Autodesk Inventor part; units mm, degrees
ref_plane "Work Plane1" through (104.775, 0, 0) normal (0, 0, -1) x (1, 0, 0)
ref_plane "YZ Plane" through (0, 0, 0) normal (1, 0, 0) x (0, 1, 0)
ref_plane "XZ Plane" through (0, 0, 0) normal (0, 1, 0) x (-1, 0, 0)
sketch "Sketch1" plane through (0, 0, 0) normal (0, 0, 1) x (1, 0, 0)
  line L0 (15.875, 0) -> (15.875, 2.0828)
  line L1 (15.875, 2.0828) -> (4.8293, 2.0828)
  line L2 (4.8293, 2.0828) -> (2.8448, 2.0828)
  line L3 (0, 3.9497) -> (0, 1.3785)
  line L4 (0, 1.3785) -> (1.9304, 1.3785)
  line L5 (1.9304, 1.3785) -> (2.7263, 0)
  line L6 (2.7263, 0) -> (15.875, 0)
  line L7 (0, 3.9497) -> (0.6972, 3.9497)
  line L8 (0.6972, 3.9497) -> (2.8448, 2.0828)
  line L9 (2.8448, 2.0828) -> (2.8448, 2.0828)
  line L10 (4.8293, 2.0828) -> (2.8448, 2.0828) construction
  line L11 (2.8448, 2.0828) -> (2.8448, 2.0828)
  line L12 (-3.175, 0) -> (19.05, 0)
  line L13 (0, -0.7899) -> (0, 4.7396)
  dimension "d0" = 15.875
  dimension "d1" = 11.0457
  dimension "d2" = 1.9304
  dimension "d3" = 4.1656
  dimension "d6" = 2.8448
  dimension "d7" = 41
  dimension "d8" = 2.757
  dimension "d9" = 60
  dimension "d10" = 7.8994
  dimension "d11" = 4.1656
  dimension "d12" = 1.9845
revolve "Body" add sketch "Sketch1" angle 360 about axis through (2.7263, 0, 0) along (1, 0, 0) contours L6 L5 L4 L3 L7 L8 L2 L1 L0
sketch "Sketch2" plane through (0, 0, 0) normal (-1, 0, 0) x (0, 0, 1)
  circle A0 centre (0, 0) radius 1.3785
  line L0 (0, -5.5296) -> (0, 5.5296)
  line L1 (-5.5296, 0) -> (5.5296, 0)
  line L2 (1.3785, 0) -> (0.6892, -1.1938)
  line L3 (0.6892, -1.1938) -> (-0.6892, -1.1938)
  line L4 (-0.6892, -1.1938) -> (-1.3785, 0)
  line L5 (-1.3785, 0) -> (-0.6892, 1.1938)
  line L6 (-0.6892, 1.1938) -> (0.6892, 1.1938)
  line L7 (0.6892, 1.1938) -> (1.3785, 0)
  point P0 (0, 1.3785)
extrude "Slot" add sketch "Sketch2" against normal up to next contours L7 A0 | A0 L2 | L6 L0 A0 | A0 L0 L3 | L0 L6 A0 | A0 L3 L0 | L4 A0 | A0 L5
thread "Thread"
chamfer "Chamfer1" distance 0.4724 distance2 0.9449 1 edges at (15.875, -2.0828, 0) measured on face at (15.875, 0.3944, 0.7269)
ref_plane "Work Plane1" through (104.775, 0, 0) normal (0, 0, -1) x (1, 0, 0)
equation "\"d15\" = GEL"
equation "\"d17\" = -0.5 * SPD + 0.5 * GD"
equation "\"d18\" = GUL"
equation "\"d0\" = NLG"
equation "\"d1\" = GEL"
equation "\"d2\" = INTI"
equation "\"d3\" = GD"
equation "\"d6\" = KOH"
equation "\"d7\" = 0.5 * SEWI"
equation "\"d8\" = 1.1547 * SW"
equation "\"d10\" = KOD"
equation "\"d11\" = BDM"
equation "\"d12\" = GAL"
equation "\"NLG\" = 15.875"
equation "\"INTI\" = 1.9304"
equation "\"GEL\" = 11.0457"
equation "\"GAL\" = 1.9845"
equation "\"KOH\" = 2.8448"
equation "\"KOD\" = 7.8994"
equation "\"GUL\" = 0.94488"
equation "\"SPD\" = 3.22072"
equation "\"BDM\" = NND"
equation "\"GD\" = NND"
equation "\"SEWI\" = 82deg"
equation "\"SW\" = 2.3876"
equation "\"TOA\" = 30deg"
equation "\"GD1\" = SPD"
equation "\"THREADDIA\" = 4.1656"
equation "\"HHPTC\" = 0.79375"
equation "\"NND\" = 4.1656"
equation "\"E0\" = 1.155 * SW"
properties part number "ANSI B18.3 - 8-32 UNC x 0.625" material "Steel, Mild"
Input: part model. Units: mm. Frame: model coordinates. A direction names the side the tool comes from. Give positions to 0.01 mm unless a question says otherwise; leave off trailing zeros. Loops run counter-clockwise (first coordinate to the right, second up) from the corner with the lowest first, then second, coordinate; pieces in that order, holes last. Notation, with made-up numbers: M 57.5,61.25 L 90.5,61.25 A10 ccw 90.5,76.25 Z; hole C 22,86.25 d8. An arc over 180 degrees is marked long. Answer as CSV lines item,"result". Start each with the question number.
1. Section A-A on x = 6. Return loops of the section in (y, z).
2. Line query: L1, parallel to X at y = 1.5, z = -3; L2, parallel to Z at x = 9.25, y = 0; L3, parallel to X at y = 1.75, z = 2.5. Output: solid intervals per line, ascending.
3. Pull-direction query (Z, two-part tool) for faces 4 (the face through (1.004, -0.605, -1.029)), 5 (the face through (2.71, -0.477, 2.147)), 6 (the face through (15.875, 0, 0)); classes: released by +Z, released by -Z, zero draft, split by the parting line, or undercut.
4. Pin query (flat end, axial travel): P1, Ø4, axis at x = 8, z = 2.5, coming from the +Y side; P2, Ø1.5, axis at y = 3, z = 2.5, coming from the +X side; P3, Ø1.5, axis at x = 12, y = -2, coming from the -Z side. Return the tip coordinate at first contact, or that it passes through.
5. Reachability of faces 1 (the face through (0.353, -3.946, 0.174)), 2 (the face through (1, 1.194, 0)), 3 (the face through (8.803, 1.987, -0.626)) from +Z, -Z, +X, -X, +Y, -Y: full face, straight path, thin tool, end or side. Return the list, or none.
Computed values:
1,outline,"C 0,0 d4.17"
2,L1,"x = 0 to 1.38"
2,L2,"z = -2.08 to 2.08"
2,L3,"x = 0 to 1.73"
3,face 4,"undercut"
3,face 5,"split by the parting line"
3,face 6,"zero draft"
4,P1,"stops at y = 2.02"
4,P2,"stops at x = 1.61"
4,P3,"stops at z = -1.67"
5,face 1,"+X, -X"
5,face 2,"-X"
5,face 3,"+X"
